from build123d import *

# Parameters (mm, degrees)
SKETCH_C_W          = 250
SKETCH_C_H          = 70
BOSS_EXTRUDE1_DEPTH = 5
SKETCH2_W           = 250
SKETCH2_H           = 5
BOSS_EXTRUDE2_DEPTH = 120
SKETCH3_W           = 15
SKETCH3_H           = 10
CUT_EXTRUDE1_DEPTH  = 120
SKETCH4_W           = 140
SKETCH4_H           = 50
CUT_EXTRUDE2_DEPTH  = 5
SKETCH5_W           = 250
SKETCH5_H           = 70
BOSS_EXTRUDE3_DEPTH = 5


with BuildPart() as part:
    # Sketch C → Boss-Extrude1 (new body)
    with BuildSketch(Plane(origin=(0, 0, 0), x_dir=(1, 0, 0), z_dir=(0, 1, 0))):
        with Locations((125, 35)):
            Rectangle(SKETCH_C_W, SKETCH_C_H)
    extrude(amount=BOSS_EXTRUDE1_DEPTH)

    # Sketch2 → Boss-Extrude2 (add)
    with BuildSketch(Plane(origin=(0, 5, 0), x_dir=(1, 0, 0), z_dir=(0, 1, 0))):
        with Locations((125, 67.5)):
            Rectangle(SKETCH2_W, SKETCH2_H)
    extrude(amount=BOSS_EXTRUDE2_DEPTH)

    # Sketch3 → Cut-Extrude1 (cut)
    with BuildSketch(Plane.XY.offset(-65)):
        with Locations((98.873250263, 101.586143008)):
            Rectangle(SKETCH3_W, SKETCH3_H)
        Polygon((40.509305923, 85.05481861), (80.454487313, 82.96138036), (82.657638013, 125), (42.602744173, 125), align=None)
    extrude(amount=-CUT_EXTRUDE1_DEPTH, mode=Mode.SUBTRACT)

    # Sketch4 → Cut-Extrude2 (cut)
    with BuildSketch(Plane.XZ):
        with Locations((70, -25)):
            Rectangle(SKETCH4_W, SKETCH4_H)
    extrude(amount=-CUT_EXTRUDE2_DEPTH, mode=Mode.SUBTRACT)

    # Sketch5 → Boss-Extrude3 (add)
    with BuildSketch(Plane(origin=(0, 130, 0), x_dir=(1, 0, 0), z_dir=(0, 1, 0))):
        with Locations((125, 35)):
            Rectangle(SKETCH5_W, SKETCH5_H)
    extrude(amount=-BOSS_EXTRUDE3_DEPTH)

    # Mirror3: part across plane


with BuildPart() as part_1:
    add(part.part)
    add(part.part.mirror(Plane.XY))


solid = part_1.part
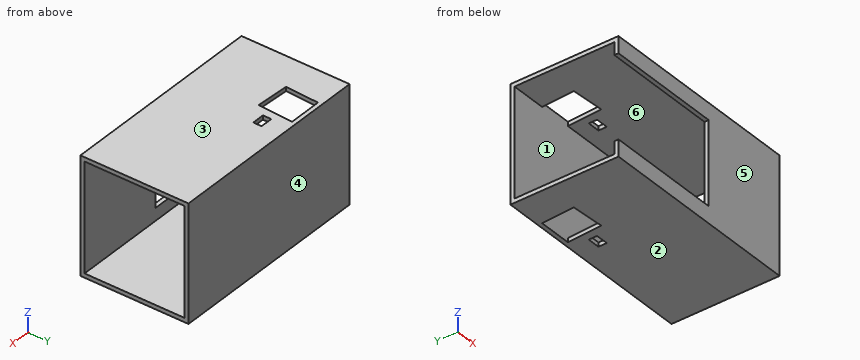
Can you work these out from the model? Positions are in its coordinate system, mm. Face numbers are marked on the shaded views. A direction names the side the tool comes from. Coordinates: 2 decimals unless noted, no trailing zeros. Loops run counter-clockwise (first coordinate to the right, second up) from the corner with the lowest first, then second, coordinate; pieces in that order, holes last. Notation, with made-up numbers: (-4.5, 49.25) - (15.5, 49.25) arc R28 cw to (15.5, 88.25) - close; hole circle Ø6 at (42, 38). An arc over 180 degrees is marked (long way). Put each result on its own line as item: value. Start each with the question number.
Item 1: Suppose I cut it at A-A (y = 22). Please give me the cut outline in (x, z), and give its area (3 significant figures).
Item 2: Suppose I cut it at B-B (x = 94). Please give me the cut outline in (y, z).
Item 3: If I drill on line 1 along Z through (x, y) = (151, 28.5); line 2 along Y through (x, z) = (25.5, -62.5); line 3 along Y through (x, z) = (85, 16.5), over which ranges is the centre line in solid material (lowest first)?
Item 4: Suppose I cut it at C-C (z = -39). Please give me the cut outline in (x, y).
Item 5: Which directions (+Z, -Z, +X, -X, +Y, -Y) give clear straight access to the entire face, cutting with the end or side of a thin tool? Please do the marked faces 5 and 6.
Item 6: If we mould it in two halves opening along Z, with no side actions, what happens to the marked faces 1, 2, 3 and 4? For each: +Z half, -Z half, draft (parallel to the pull), parting line (faces both ways), or undercut.
Item 7: For pin 1 (5.5 mm diameter, centred on y = 2.5, z = 11, fed in from -X); pin 2 (3 mm diameter, centred on x = 25.5, z = -17, fed in from -Y), each with a flat end and sliding along its axis, tell me the tip position at first contact or that it passes through.
Item 8: Suppose I cut it at D-D (x = 233.5). Please give me the cut outline in (y, z).
Here are the results:
1. outline: (0, -70) - (250, -70) - (250, -65) - (0, -65) - close; (0, 65) - (250, 65) - (250, 70) - (0, 70) - close
1. area: 2,500 mm²
2. outline: (0, -70) - (96.59, -70) - (96.59, -65) - (5, -65) - (5, -50) - (0, -50) - close; (0, 50) - (5, 50) - (5, 65) - (96.59, 65) - (96.59, 70) - (0, 70) - close; (106.59, -70) - (130, -70) - (130, 70) - (106.59, 70) - (106.59, 65) - (125, 65) - (125, -65) - (106.59, -65) - close
3. line 1: -70 to -65, 65 to 70
3. line 2: 0 to 5, 125 to 130
3. line 3: 125 to 130
4. outline: (0, 125) - (250, 125) - (250, 130) - (0, 130) - close; (140, 0) - (250, 0) - (250, 5) - (140, 5) - close
5. face 5: +Z, -Z, +X, -X, -Y
5. face 6: +X, -X
6. face 1: undercut
6. face 2: -Z half
6. face 3: +Z half
6. face 4: draft
7. pin 1: x = 140
7. pin 2: y = 125
8. outline: (0, -70) - (130, -70) - (130, 70) - (0, 70) - close; hole (5, -65) - (125, -65) - (125, 65) - (5, 65) - close
